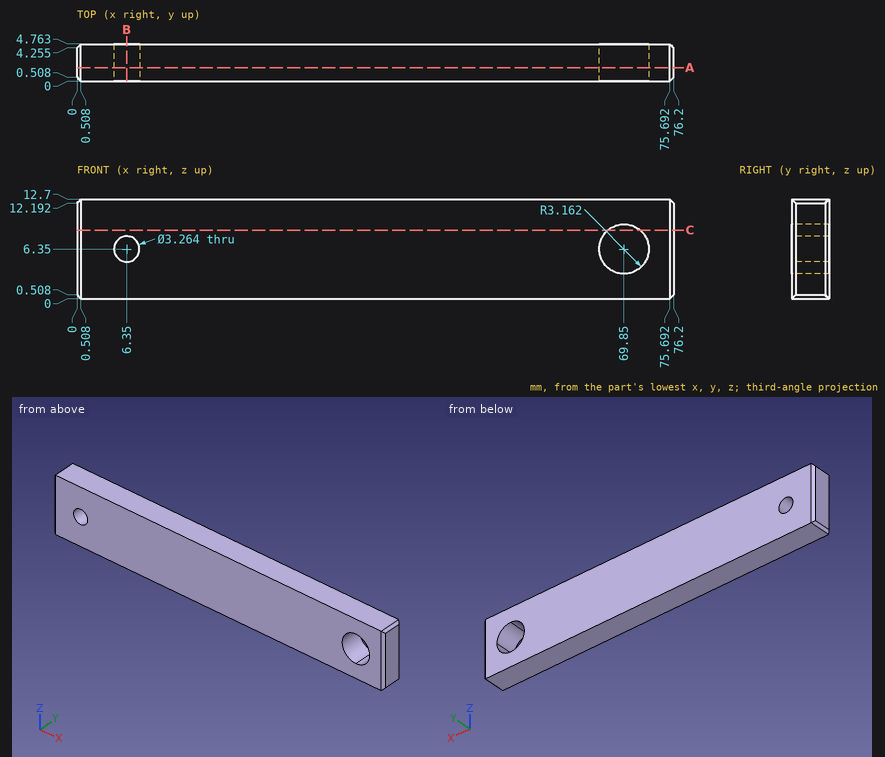
Input: dimensioned drawing with shaded views. Units: mm. Origin: part minimum x, y, z. Give positions to 0.01 mm unless a question says otherwise; leave off trailing zeros. Loops run counter-clockwise (first coordinate to the right, second up) from the corner with the lowest first, then second, coordinate; pieces in that order, holes last. Notation, with made-up numbers: M 9.5,1 L 27.5,1 A26 cw 27.5,32 Z; hole C 47.5,74.5 d5. An arc over 180 degrees is marked long. Put each result on its own line as item: value.
1) Material intervals for L1, parallel to X at y = 3.4, z = 6.25; L2, parallel to Z at x = 6.35, y = 1.55; L3, parallel to X at y = 0.5, z = 6 (1 decimal), sorted ascending. Write a range as from..to.
Computed values:
L1: x = 0..4.72, 7.98..66.69, 73.01..76.2
L2: z = 0..4.72, 7.98..12.7
L3: x = 0..4.8, 7.9..66.7, 73..76.2
2) Cut plane A-A, the plane y = 1.75. Give the number of separate pieces and of enclosed holes in the cut face.
Computed values:
separate pieces: 1
enclosed holes: 2
3) Cut plane B-B, the plane x = 6.35. Return the cut outline in (y, z).
Computed values:
outline: M 0,0 L 4.76,0 L 4.76,4.72 L 0,4.72 Z; M 0,7.98 L 4.76,7.98 L 4.76,12.7 L 0,12.7 Z
4) Cut plane C-C, the plane z = 8.75. Return the cut outline in (x, y) (1 decimal).
Computed values:
outline: M 0,0.5 L 0.5,0 L 67.8,0 L 67.8,4.8 L 0.5,4.8 L 0,4.3 Z; M 71.9,0 L 75.7,0 L 76.2,0.5 L 76.2,4.3 L 75.7,4.8 L 71.9,4.8 Z
